Autodesk Inventor part; units mm, degrees
ref_plane "YZ Plane" through (0, 0, 0) normal (1, 0, 0) x (0, 1, 0)
ref_plane "XZ Plane" through (0, 0, 0) normal (0, 1, 0) x (-1, 0, 0)
ref_plane "XY Plane" through (0, 0, 0) normal (0, 0, 1) x (1, 0, 0)
sketch "Boceto1" plane through (0, 0, 0) normal (0, 0, 1) x (1, 0, 0)
  circle A0 centre (0, 0) radius 57.15
  circle A1 centre (101.6, 0) radius 44.45
  circle A2 centre (-31.75, 47.519) radius 11.1125
  circle A3 centre (-31.75, -47.519) radius 11.1125
  circle A4 centre (114.3, 42.5971) radius 11.1125
  circle A5 centre (114.3, -42.5971) radius 11.1125
  line L0 (7.1437, 56.7018) -> (107.1562, 44.1014)
  circle A6 centre (44.45, 52.0016) radius 11.1125
  line L1 (7.1437, -56.7018) -> (107.1562, -44.1014)
  circle A7 centre (44.45, -52.0016) radius 11.1125
  dimension "d0" = 114.3
  dimension "d1" = 88.9
  dimension "d2" = 203.2
  dimension "d3" = 22.225
  dimension "d4" = 22.225
  dimension "d7" = 22.225
  dimension "d8" = 22.225
  dimension "d11" = 22.225
  dimension "d13" = 0
  dimension "d14" = 22.225
  dimension "d27" = 12.7
  dimension "d28" = 12.7
  dimension "d29" = 44.45
  dimension "d30" = 44.45
  dimension "d31" = 31.75
  dimension "d32" = 31.75
extrude "Extrusión1" add sketch "Boceto1" along normal blind 5
sketch "Boceto2" plane through (0, 0, 5) normal (0, 0, 1) x (1, 0, 0)
  arc A0 (-21.9537, 52.7651) -> (-40.3458, 40.4764) centre (-31.75, 47.519) ccw
  circle A1 centre (-31.75, 47.519) radius 4.7625
  arc A2 (-40.3458, -40.4764) -> (-21.9537, -52.7651) centre (-31.75, -47.519) ccw
  circle A3 centre (-31.75, -47.519) radius 4.7625
  arc A4 (33.4247, -53.3907) -> (55.4753, -50.6125) centre (44.45, -52.0016) ccw
  circle A5 centre (44.45, -52.0016) radius 4.7625
  arc A6 (55.4753, 50.6125) -> (33.4247, 53.3907) centre (44.45, 52.0016) ccw
  circle A7 centre (44.45, 52.0016) radius 4.7625
  arc A8 (124.4689, 38.1158) -> (103.3657, 44.5789) centre (114.3, 42.5971) ccw
  circle A9 centre (114.3, 42.5971) radius 4.7625
  arc A10 (103.3657, -44.5789) -> (124.4689, -38.1158) centre (114.3, -42.5971) ccw
  circle A11 centre (114.3, -42.5971) radius 4.7625
  point P0 (0, 0)
  dimension "d18" = 9.525
  dimension "d19" = 9.525
  dimension "d20" = 9.525
  dimension "d21" = 9.525
  dimension "d22" = 9.525
  dimension "d23" = 9.525
extrude "Extrusión2" cut sketch "Boceto2" against normal up to surface (5 mm away)
fillet "Empalme1" radius 6.35 12 edges at (-21.9537, -52.7651, 2.5) (-40.3458, -40.4764, 2.5) (33.4247, -53.3907, 2.5) (55.4753, -50.6125, 2.5) (124.4689, -38.1158, 2.5) (-40.3458, 40.4764, 2.5) (-21.9537, 52.7651, 2.5) (33.4247, 53.3907, 2.5) (55.4753, 50.6125, 2.5) (103.3657, 44.5789, 2.5) (124.4689, 38.1158, 2.5) (103.3657, -44.5789, 2.5)
sketch "Boceto3" plane through (0, 0, 0) normal (0, 0, -1) x (-1, 0, 0)
  circle A0 centre (0, 0) radius 7.1437
  circle A1 centre (0, -45) radius 6.35
  circle A2 centre (0, 45) radius 6.35
  line L0 (0, -45) -> (0, 0)
  line L1 (0, 0) -> (0, 45)
  dimension "d33" = 14.2875
  dimension "d34" = 12.7
  dimension "d35" = 12.7
  dimension "d36" = 45
  dimension "d37" = 45
extrude "Extrusión3" cut sketch "Boceto3" against normal up to surface (5 mm away)
sketch "Boceto4" plane through (0, 0, 5) normal (0, 0, 1) x (1, 0, 0)
  circle A0 centre (93.4212, 0) radius 6.35
  line L0 (65.4212, -28) -> (121.4212, -28)
  line L1 (121.4212, -28) -> (121.4212, 28)
  line L2 (121.4212, 28) -> (65.4212, 28)
  line L3 (65.4212, 28) -> (65.4212, -28)
  line L4 (69.6712, -23.75) -> (117.1712, -23.75)
  line L5 (117.1712, -23.75) -> (117.1712, 23.75)
  line L6 (117.1712, 23.75) -> (69.6712, 23.75)
  line L7 (69.6712, 23.75) -> (69.6712, -23.75)
  circle A1 centre (74.8306, -23.75) radius 2.7781
  circle A2 centre (112.0118, -23.75) radius 2.7781
  circle A3 centre (122.3306, -23.75) radius 2.7781
  circle A4 centre (64.5118, -23.75) radius 2.7781
  line L8 (64.5118, -26.5281) -> (74.8306, -26.5281)
  line L9 (64.5118, -20.9719) -> (74.8306, -20.9719)
  line L10 (112.0118, -26.5281) -> (122.3306, -26.5281)
  line L11 (122.3306, -20.9719) -> (112.0118, -20.9719)
  circle A5 centre (74.8306, 23.75) radius 2.7781
  circle A6 centre (64.5118, 23.75) radius 2.7781
  line L12 (64.5118, 20.9719) -> (74.8306, 20.9719)
  line L13 (64.5118, 26.5281) -> (74.8306, 26.5281)
  circle A7 centre (112.0118, 23.75) radius 2.7781
  circle A8 centre (122.3306, 23.75) radius 2.7781
  line L14 (112.0118, 20.9719) -> (122.3306, 20.9719)
  line L15 (112.0118, 26.5281) -> (122.3306, 26.5281)
  circle A9 centre (98.5806, 0) radius 6.35
  circle A10 centre (88.2618, 0) radius 6.35
  line L16 (98.5806, 6.35) -> (88.2618, 6.35)
  line L17 (98.5806, -6.35) -> (88.2618, -6.35)
  point P0 (0, 0)
  dimension "d40" = 12.7
  dimension "d41" = 56
  dimension "d42" = 56
  dimension "d43" = 28
  dimension "d44" = 28
  dimension "d45" = 0
  dimension "d46" = 93.4212
  dimension "d47" = 47.5
  dimension "d48" = 47.5
  dimension "d49" = 23.75
  dimension "d50" = 23.75
  dimension "d57" = 5.5563
  dimension "d58" = 5.1594
  dimension "d59" = 5.5563
  dimension "d60" = 5.5563
  dimension "d61" = 5.1594
  dimension "d62" = 5.1594
  dimension "d63" = 5.5563
  dimension "d64" = 5.1594
  dimension "d65" = 0
  dimension "d66" = 5.5563
  dimension "d67" = 5.5563
  dimension "d68" = 5.1594
  dimension "d69" = 5.1594
  dimension "d70" = 0
  dimension "d71" = 5.5563
  dimension "d72" = 5.5563
  dimension "d73" = 5.1594
  dimension "d74" = 5.1594
  dimension "d75" = 0
  dimension "d78" = 12.7
  dimension "d79" = 12.7
  dimension "d80" = 5.1594
  dimension "d81" = 5.1594
extrude "Extrusión4" cut sketch "Boceto4" against normal up to next contours A0 A9 A10 | A0 A9 | A9 A10 A0 | A0 L16 A9 | A9 L17 A0 | A0 A10 A9 | A0 A10 L16 | A10 A9 | A9 A10 A0 | L17 A10 A0 | A0 A10 | L8 A4 L3 | L3 A4 L9 L7 L4 A1 L8 | L10 A2 L4 L5 L11 L1 A3 | L1 A3 L10 | A4 L3 | L3 A4 | A1 L4 | A3 L1 | L1 A3 | A2 L4 | A4 L9 L3 | L4 A1 | L4 L7 L9 A1 | L1 L11 A3 | A2 L11 L5 L4 | L4 A2 | L12 A6 L3 | L3 A6 L13 A5 L6 L7 L12 | L14 L5 L6 A7 L15 L1 A8 | L1 A8 L14 | A6 L3 | L3 A6 | L7 L6 A5 L12 | A8 L1 | L1 A8 | L14 A7 L6 L5 | A6 L13 L3 | A5 L6 | L1 L15 A8 | A7 L6 | A5 L6 | L6 A7
sketch "Boceto5" plane through (0, 0, 5) normal (0, 0, 1) x (1, 0, 0)
  line L0 (50.8, -13.7453) -> (-50.8, -13.7453)
  line L1 (-50.8, -13.7453) -> (-50.8, -114.3)
  line L2 (-50.8, -114.3) -> (50.8, -114.3)
  line L3 (50.8, -114.3) -> (50.8, -13.7453)
  arc A0 (7.1437, 56.7018) -> (-17.8783, 54.2816) centre (0, 0) ccw
  arc A1 (7.1437, 56.7018) -> (-17.8783, 54.2816) centre (0, 0) ccw
  line L4 (0, 57.15) -> (7.6634, 57.15)
  arc A2 (127.9228, -35.8178) -> (127.9228, 35.8178) centre (101.6, 0) ccw
  line L5 (146.05, 0) -> (146.05, -27.5116)
  dimension "d82" = 101.6
  dimension "d84" = 171.45
  dimension "d85" = 95.25
extrude "Extrusión5" add sketch "Boceto5" against normal up to surface (5 mm away)
extrude "Extrusión6" cut sketch "Boceto2" against normal up to next contours A3 | A5
sketch "Boceto7" plane through (0, 0, 5) normal (0, 0, 1) x (1, 0, 0)
  circle A0 centre (31.75, -69.85) radius 4.3656
  circle A1 centre (31.75, -76.2) radius 4.3656
  line L0 (50.8, -114.3) -> (50.8, -61.1211)
  line L1 (-50.8, -114.3) -> (50.8, -114.3)
  line L2 (36.1156, -69.85) -> (36.1156, -76.2)
  line L3 (27.3844, -69.85) -> (27.3844, -76.2)
  circle A2 centre (31.75, -95.25) radius 4.3656
  circle A3 centre (31.75, -101.6) radius 4.3656
  line L4 (36.1156, -95.25) -> (36.1156, -101.6)
  line L5 (27.3844, -101.6) -> (27.3844, -95.25)
  point P0 (0, 0)
  dimension "d90" = 8.7312
  dimension "d91" = 8.7312
  dimension "d92" = 19.05
  dimension "d93" = 44.45
  dimension "d94" = 38.1
  dimension "d95" = 0
  dimension "d96" = 8.7312
  dimension "d97" = 8.7312
  dimension "d98" = 19.05
  dimension "d99" = 19.05
  dimension "d100" = 12.7
  dimension "d101" = 0
extrude "Extrusión7" cut sketch "Boceto7" against normal up to next
mirror "Simetría1" about plane through (0, 0, 0) normal (1, 0, 0) of "Extrusión7"
fillet "Empalme2" radius 6.35 4 edges at (-50.8, -26.1817, 2.5) (-50.8, -114.3, 2.5) (50.8, -61.1211, 2.5) (50.8, -114.3, 2.5)
extrude "Extrusión8" cut sketch "Boceto3" against normal up to next contours A1
equation "\"d16\" = t"
equation "\"d18\" = Q"
equation "\"d19\" = Q"
equation "\"d20\" = Q"
equation "\"d21\" = Q"
equation "\"d22\" = Q"
equation "\"d23\" = Q"
equation "\"d33\" = DF"
equation "\"d34\" = NF"
equation "\"d35\" = NF"
equation "\"d40\" = DM"
equation "\"d41\" = AM"
equation "\"d42\" = AM"
equation "\"d43\" = 0.5 * AM"
equation "\"d44\" = 0.5 * AM"
equation "\"d47\" = BM"
equation "\"d48\" = BM"
equation "\"d49\" = 0.5 * BM"
equation "\"d50\" = 0.5 * BM"
equation "\"d57\" = NM"
equation "\"d59\" = NM"
equation "\"d60\" = NM"
equation "\"d63\" = NM"
equation "\"d66\" = NM"
equation "\"d67\" = NM"
equation "\"d71\" = NM"
equation "\"d72\" = NM"
equation "\"d78\" = DM"
equation "\"d79\" = DM"
equation "\"d90\" = DH"
equation "\"d91\" = DH"
equation "\"d96\" = DH"
equation "\"d97\" = DH"
equation "\"t\" = 5"
equation "\"Q\" = 9.525"
equation "\"DF\" = 14.2875"
equation "\"NF\" = 12.7"
equation "\"DM\" = 12.7"
equation "\"NM\" = 5.55625"
equation "\"CM\" = 93.4212"
equation "\"AM\" = 56"
equation "\"BM\" = 47.5"
equation "\"DH\" = 8.73125"
properties part number "CAR REDUCTION PLATE II"
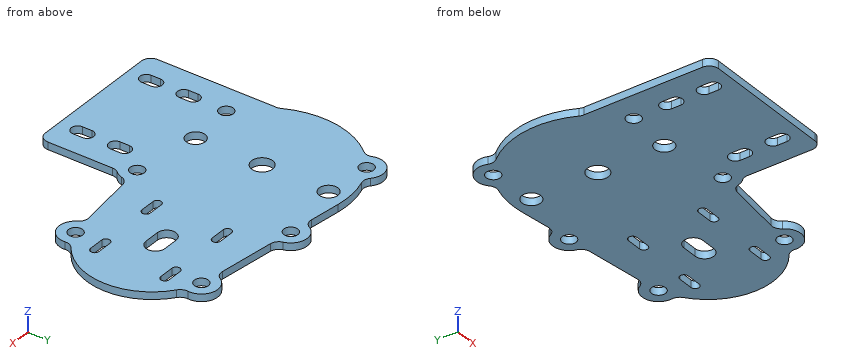
Here's how the part is built. I have some questions about the finished solid (model axes, mm). Give positions to 0.01 mm unless a question says otherwise; leave off trailing zeros. Order: outer loops, then holes, each group sorted by start corner. A loop starts at its lowest first (then second) coordinate and runs counter-clockwise, first axis right, second up. Notation, with made-up numbers: (50, 2) -> (57, 2) arc R19 cw to (57, 8) -> close; hole circle Ø5 at (68, 52.25). An arc over 180 degrees is marked (long way). Use a Markdown table: item, result. Add a question column.
Item 1: I need wall thicknesses on line 1 (X direction, y = -72.5, z = 2.4); line 2 (Y direction, x = 44.45, z = 2.4); line 3 (Y direction, x = -31.75, z = 3.8). Which ranges of each line are inside material? Lowest first, please.
Item 2: Imagine slicing it at C-C on y = 0. Please give me the cut outline in (x, z).
Item 3: Imagine slicing it at D-D on z = 1.65. Give the number of separate pieces and of enclosed holes in the cut face, plus the area to 3 significant figures.
Item 4: Imagine slicing it at B-B on x = 0. Please give me the cut outline in (y, z).
Item 5: Imagine slicing it at A-A on y = -74. Please give me the cut outline in (x, z), plus the area to 3 significant figures.
Item 6: Will these pins go through, and if not, where does the flat tip stop? pin 1 (11 mm diameter, centred on x = 114.3, y = -42.6, fed in from -Z); pin 2 (2.5 mm diameter, centred on y = -72, z = 3.5, fed in from -X); pin 3 (2.5 mm diameter, centred on x = 119.5, z = 3.5, fed in from +Y); pin 4 (10 mm diameter, centred on x = 0, y = 45, fed in from -Z).
Data:
| question | item | result |
|---|---|---|
| 1 | line 1 | x = -50.8 to -36.12, -27.38 to 27.38, 36.12 to 50.8 |
| 1 | line 2 | y = -114.3 to -56.76, -47.24 to 47.24, 56.76 to 63.11 |
| 1 | line 3 | y = -114.3 to -105.97, -90.88 to -80.57, -65.48 to -52.28, -42.76 to 42.76, 52.28 to 58.63 |
| 2 | outline | (-57.15, 0) -> (-7.14, 0) -> (-7.14, 5) -> (-57.15, 5) -> close; (7.14, 0) -> (81.91, 0) -> (81.91, 5) -> (7.14, 5) -> close; (104.93, 0) -> (146.05, 0) -> (146.05, 5) -> (104.93, 5) -> close |
| 3 | separate pieces | 1 |
| 3 | enclosed holes | 18 |
| 3 | area | 24,000 mm² |
| 4 | outline | (-114.3, 0) -> (-51.35, 0) -> (-51.35, 5) -> (-114.3, 5) -> close; (-38.65, 0) -> (-7.14, 0) -> (-7.14, 5) -> (-38.65, 5) -> close; (7.14, 0) -> (38.65, 0) -> (38.65, 5) -> (7.14, 5) -> close; (51.35, 0) -> (57.15, 0) -> (57.15, 5) -> (51.35, 5) -> close |
| 5 | outline | (-50.8, 0) -> (-36.12, 0) -> (-36.12, 5) -> (-50.8, 5) -> close; (-27.38, 0) -> (27.38, 0) -> (27.38, 5) -> (-27.38, 5) -> close; (36.12, 0) -> (50.8, 0) -> (50.8, 5) -> (36.12, 5) -> close |
| 5 | area | 421 mm² |
| 6 | pin 1 | stops at z = 0 |
| 6 | pin 2 | stops at x = -50.8 |
| 6 | pin 3 | stops at y = 52.98 |
| 6 | pin 4 | passes through |
